Input: dimensioned drawing with shaded views. Units: mm. Origin: part minimum x, y, z. A direction names the side the tool comes from. Coordinates: 2 decimals unless noted, no trailing zeros. Order: outer loops, then holes, each group sorted by start corner. A loop starts at its lowest first (then second) coordinate and runs counter-clockwise, first axis right, second up.
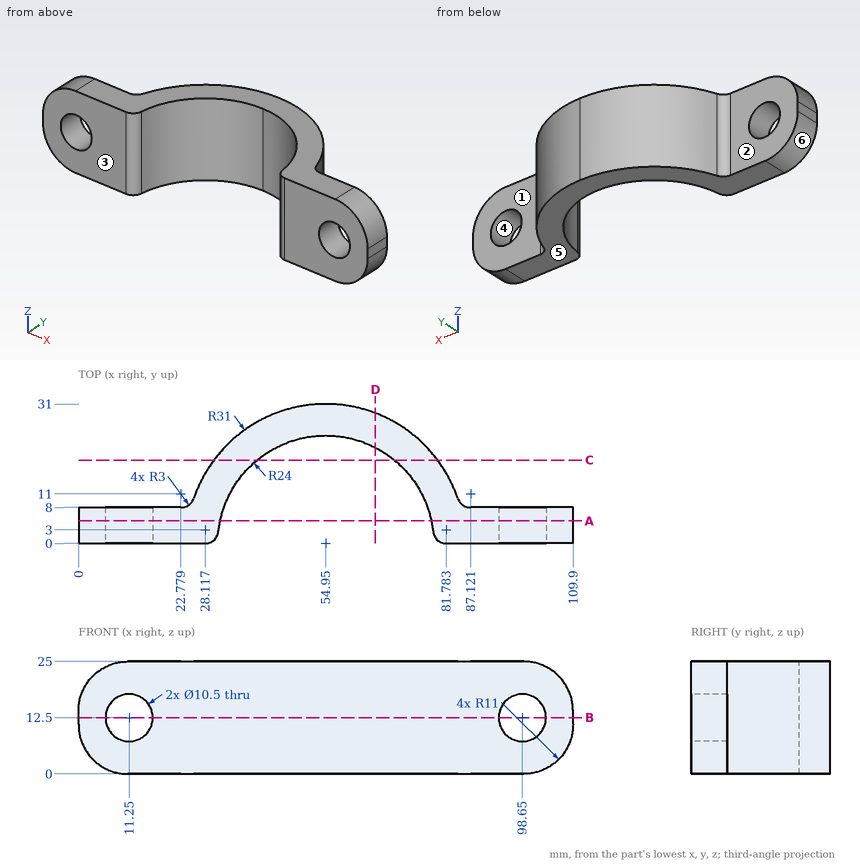
1. Section query B-B, the plane z = 12.5. Output: boundary loops of the cut face in (x, y).
2. Section query C-C, the plane y = 18.5. Output: boundary loops of the cut face in (x, z) (1 decimal), plus the area to 3 significant figures.
3. Section query D-D, the plane x = 66. Output: boundary loops of the cut face in (y, z) (1 decimal).
4. Material intervals for line 1 along Z through (x, y) = (11.25, 3.75); line 2 along X through (y, z) = (5, 2.25) (1 decimal); line 3 along Y through (x, z) = (9, 4.25), sorted ascending.
5. Draft query along X for the marked faces 4, 5 and 6. Return one class per face: +X half, -X half, draft (parallel to the pull), parting line (faces both ways), or undercut.
6. Contact query for flat-ended pins moving along their axis: P1, Ø13.5, axis at x = 98.65, z = 12.5, coming from the +Y side; P2, Ø1.5, axis at y = 5, z = 7.5, coming from the -X side; P3, Ø2, axis at x = 29.5, z = 20, coming from the -Y side (1 decimal); P4, Ø4, axis at y = 3.5, z = 14.5, coming from the -X side. Output: stop coordinate, or through.
7. Section query A-A, the plane y = 5. Output: boundary loops of the cut face in (x, z), plus the area to 3 significant figures.
8. Access query for the marked faces 1, 2 and 3. Directions: +Z, -Z, +X, -X, +Y, -Y. A direction counts if a zero-diameter tool reaches every point of the face in a straight line with its end or side. Return the directions, or none.
Answer key:
1. outline: (0, 0) - (6, 0) - (6, 8) - (0, 8) - close; (16.5, 0) - (28.12, 0) arc R3 ccw to (31.1, 2.67) arc R24 cw to (54.95, 24) arc R24 cw to (78.8, 2.67) arc R3 ccw to (81.78, 0) - (93.4, 0) - (93.4, 8) - (87.12, 8) arc R3 cw to (84.28, 10.03) arc R31 ccw to (25.62, 10.03) arc R3 cw to (22.78, 8) - (16.5, 8) - close; (103.9, 0) - (109.9, 0) - (109.9, 8) - (103.9, 8) - close
2. outline: (30.1, 0) - (39.7, 0) - (39.7, 25) - (30.1, 25) - close; (70.2, 0) - (79.8, 0) - (79.8, 25) - (70.2, 25) - close
2. area: 479 mm2
3. outline: (21.3, 0) - (29, 0) - (29, 25) - (21.3, 25) - close
4. line 1: z = 0 to 7.25, 17.75 to 25
4. line 2: x = 4.3 to 31.5, 78.4 to 105.6
4. line 3: y = 0 to 8
5. face 4: undercut
5. face 5: draft
5. face 6: -X half
6. P1: stops at y = 8
6. P2: stops at x = 0.35
6. P3: stops at y = 0
6. P4: stops at x = 0
7. outline: (0, 11) arc R11 ccw to (11, 0) - (31.48, 0) - (31.48, 25) - (11, 25) arc R11 ccw to (0, 14) - close; (78.42, 0) - (98.9, 0) arc R11 ccw to (109.9, 11) - (109.9, 14) arc R11 ccw to (98.9, 25) - (78.42, 25) - close; hole circle Ø10.5 at (11.25, 12.5); hole circle Ø10.5 at (98.65, 12.5)
7. area: 1,300 mm2
8. face 1: +Z, -Z, +X, +Y
8. face 2: +Z, -Z, -X, +Y
8. face 3: +Z, -Z, +X, -X, -Y
